For this review, take the finished solid that the model builds, in its own axes (mm). A direction names the side the tool comes from. Round coordinates to 2 decimals unless told otherwise and drop trailing zeros. Loops run counter-clockwise (first coordinate to the right, second up) from the corner with the lowest first, then second, coordinate; pieces in that order, holes last. Notation, with made-up numbers: (84.5, 62) -> (98.5, 62) arc R6 ccw to (98.5, 73) -> close; hole circle Ø3 at (-28, 40). An arc over 180 degrees is marked (long way). Write each question's results on one line, items separated by ' | '.
```python
from build123d import *

# Parameters (mm, degrees)
SKETCH_1_R          = 15.25
EXTRUDE_1_DEPTH     = 4
CUT_EXTRUDE_1_DEPTH = 24.002717231
EXTRUDE_3_REACH     = 33.482
SKETCH_17_W         = 11.236102528
SKETCH_17_H         = 8
SKETCH_16_R         = 1
CUT_EXTRUDE_7_DEPTH = 22.93456194
EXTRUDE_START       = 1
SKETCH_18_R         = 2.5
SKETCH_18_R_2       = 1
EXTRUDE_4_DEPTH     = 1
SKETCH_19_W         = 6
SKETCH_19_H         = 3
EXTRUDE_5_DEPTH     = 4
FILLET_1_R          = 0.5


with BuildPart() as part:
    # 草图1 → 凸台-拉伸1 (new, symmetric)
    with BuildSketch(Plane(origin=(0, 0, 0), x_dir=(1, 0, 0), z_dir=(0, 1, 0))):
        with Locations(Location((0, 0, 0), (0, 0, 270))):
            Circle(SKETCH_1_R)
    extrude(amount=EXTRUDE_1_DEPTH, both=True)

    # 草图2 → 切除-拉伸1 (cut, through all)
    with BuildSketch(Plane(origin=(0, 4, 0), x_dir=(1, 0, 0), z_dir=(0, 1, 0))):
        with BuildLine():
            Line((-12, 5.618051264), (-12, -5.618051264))
            ThreePointArc((-12, -5.618051264), (-11.175427785, -7.118448835), (-10.164275675, -8.5))
            Line((-10.164275675, -8.5), (10.164275675, -8.5))
            ThreePointArc((10.164275675, -8.5), (11.175427785, -7.118448835), (12, -5.618051264))
            Line((12, -5.618051264), (12, 5.618051264))
            ThreePointArc((12, 5.618051264), (0, 13.25), (-12, 5.618051264))
        make_face()
    extrude(amount=-CUT_EXTRUDE_1_DEPTH, mode=Mode.SUBTRACT)

    # 草图3 → 切除-旋转4 (revolve, cut)
    with BuildSketch(Plane(origin=(0, 0, 0), x_dir=(1, 0, 0), z_dir=(0, 1, 0)), mode=Mode.PRIVATE) as cut_revolve_4_sk:
        Polygon((12, 0), (12, 1.75), (14, 1.75), (14, 3), (20, 3), (20, 0), align=None)
    cut_revolve_4 = revolve(cut_revolve_4_sk.sketch.rotate(Axis((0, 0, 0), (1, 0, 0)), 180), axis=Axis((0, 0, 0), (1, 0, 0)), mode=Mode.SUBTRACT)

    # 镜向1: 切除-旋转4 across plane
    add(cut_revolve_4.mirror(Plane(origin=(0, 0, 0), x_dir=(0, 0, 1), z_dir=(1, 0, 0))), mode=Mode.SUBTRACT)

    # 草图17 → 凸台-拉伸3 (add, up to next)
    with BuildSketch(Plane.XY.offset(-12), mode=Mode.PRIVATE) as extrude_3_sk1:
        Rectangle(SKETCH_17_W, SKETCH_17_H)
    extrude_3_tool1 = extrude(extrude_3_sk1.sketch, amount=-EXTRUDE_3_REACH, mode=Mode.PRIVATE) - part.part
    add(extrude_3_tool1.solids().sort_by_distance((0, 0, -12))[0])

    # 草图16 → 切除-拉伸7 (cut, through all)
    with BuildSketch(Plane.XY):
        Circle(SKETCH_16_R)
    extrude(amount=-CUT_EXTRUDE_7_DEPTH, mode=Mode.SUBTRACT)

    # 草图18 → 凸台-拉伸4 (add)
    with BuildSketch(Plane.XY.offset(-12).offset(EXTRUDE_START)):
        Circle(SKETCH_18_R)
        Circle(SKETCH_18_R_2, mode=Mode.SUBTRACT)
    extrude(amount=-EXTRUDE_4_DEPTH)

    # 草图19 → 凸台-拉伸5 (add)
    with BuildSketch(Plane.XZ.offset(4)):
        with Locations((0, 11)):
            Rectangle(SKETCH_19_W, SKETCH_19_H)
    extrude(amount=EXTRUDE_5_DEPTH)

    # 圆角1
    fillet_1_edges = [part.edges().sort_by_distance(p)[0] for p in [
        (3, -6, 9.5),
        (3, -6, 12.5),
        (-3, -6, 12.5),
        (-3, -6, 9.5),
    ]]
    fillet(fillet_1_edges, radius=FILLET_1_R)


solid = part.part
```
1. Tool access review of faces 1 (the face through (14, 2, 0)), 2 (the face through (-0.54, -2.44, -11.49)), 3 (the face through (0, -8, 11)), 4 (the face through (-9.323, 0.056, -9.415)), 5 (the face through (-14.5, -0.1, -3)): name each direction out of +Z, -Z, +X, -X, +Y, -Y from which nothing blocks a thin tool from reaching the whole face with its end or side.
Values found:
face 1: +X | face 2: none | face 3: +Z, -Z, +X, -X, -Y | face 4: +Y, -Y | face 5: -X
2. For pin 1 (10 mm diameter, centred on x = 5, z = -4, fed in from -Y); pin 2 (4.5 mm diameter, centred on y = 0, z = 0, fed in from -X); pin 3 (8 mm diameter, centred on x = 10.5, z = 1, fed in from -Y); pin 4 (1 mm diameter, centred on x = 3, y = -1, fed in from -Z), all flat-tipped, find the tip position at first contact; note any pin that passes through.
Values found:
pin 1: passes through | pin 2: stops at x = -14 | pin 3: stops at y = -4 | pin 4: stops at z = -15.04
3. Consider section A-A (x = 0). State the section outline as (y, z) points.
Values found:
outline: (-8, 9.5) -> (-4, 9.5) -> (-4, 8.5) -> (4, 8.5) -> (4, 15.25) -> (-4, 15.25) -> (-4, 12.5) -> (-8, 12.5) -> close; (-4, -15.25) -> (-1, -15.25) -> (-1, -11) -> (-2.5, -11) -> (-2.5, -12) -> (-4, -12) -> close; (1, -15.25) -> (4, -15.25) -> (4, -12) -> (2.5, -12) -> (2.5, -11) -> (1, -11) -> close
4. Consider section B-B (z = 0). State the section outline as (x, y) points, plus the area to 3 significant figures.
Values found:
outline: (-15.25, -4) -> (-12, -4) -> (-12, -1.75) -> (-14, -1.75) -> (-14, -3) -> (-15.25, -3) -> close; (-15.25, 3) -> (-14, 3) -> (-14, 1.75) -> (-12, 1.75) -> (-12, 4) -> (-15.25, 4) -> close; (12, -4) -> (15.25, -4) -> (15.25, -3) -> (14, -3) -> (14, -1.75) -> (12, -1.75) -> close; (12, 1.75) -> (14, 1.75) -> (14, 3) -> (15.25, 3) -> (15.25, 4) -> (12, 4) -> close | area: 23.0 mm2
5. Consider section C-C (y = 0). Give the number of separate pieces and of enclosed holes in the cut face, plus the area to 3 significant figures.
Values found:
separate pieces: 3 | enclosed holes: 0 | area: 243 mm2
6. Consider section D-D (z = -7). State the section outline as (x, y) points, plus the area to 3 significant figures.
Values found:
outline: (-13.55, -4) -> (-11.25, -4) -> (-11.25, 4) -> (-13.55, 4) -> close; (11.25, -4) -> (13.55, -4) -> (13.55, 4) -> (11.25, 4) -> close | area: 36.8 mm2
7. To check wall thickness, follow probe 1 along X at (y, z) = (0, -2); probe 2 along Y at (x, z) = (0, -13); probe 3 along Y at (x, z) = (-14.6, 0). State the ranges of each line that lie inside material, in increasing order.
Values found:
probe 1: x = -14 to -12, 12 to 14 | probe 2: y = -4 to -1, 1 to 4 | probe 3: y = -4 to -3, 3 to 4
8. Draft analysis for pull direction Z (two halves, no side actions). For faces 6 (the face through (13.014, 0.67, 1.617)), 7 (the face through (0, -6, 9.5)), 8 (the face through (0, -1, -13)), 9 (the face through (14.5, -0.1, -3)), state which applies: released by +Z, released by -Z, zero draft, split by the parting line, or undercut.
Values found:
face 6: undercut | face 7: released by -Z | face 8: zero draft | face 9: undercut
